Source: CAD feature listing. Evaluate the final solid. Frame: model axes, mm. A direction names the side the tool comes from. Round coordinates to 2 decimals unless told otherwise and drop trailing zeros. Loops run counter-clockwise (first coordinate to the right, second up) from the corner with the lowest first, then second, coordinate; pieces in that order, holes last. Notation, with made-up numbers: M 60.5,2.5 L 105.5,2.5 A25 cw 105.5,29.5 Z; hole C 79,24.25 d8. An arc over 180 degrees is marked long. One line per item, written item: value.
from build123d import *

# Parameters (mm, degrees)
SALIENTE_EXTRUIR1_DEPTH = 50.8
CROQUIS2_R              = 6.5
CORTAR_EXTRUIR1_DEPTH   = 10
CROQUIS3_R              = 6.5
CORTAR_EXTRUIR2_DEPTH   = 10


with BuildPart() as part:
    # Croquis1 → Saliente-Extruir1 (new body)
    with BuildSketch(Plane(origin=(0, 0, 0), x_dir=(0, 0, -1), z_dir=(1, 0, 0))):
        Polygon((-6.31, 95.93), (0, 95.93), (0, 0), (-902.2, 0), (-902.2, 6.31), (-6.31, 6.31), align=None)
    extrude(amount=SALIENTE_EXTRUIR1_DEPTH)

    # Croquis2 → Cortar-Extruir1 (cut)
    with BuildSketch(Plane(origin=(0, 0, 0), x_dir=(-1, 0, 0), z_dir=(0, -1, 0))):
        with Locations(Location((-25.4, -885.7, 0), (0, 0, 90))):
            Circle(CROQUIS2_R)
        with Locations(Location((-25.4, -854.7, 0), (0, 0, 90))):
            Circle(CROQUIS2_R)
    extrude(amount=-CORTAR_EXTRUIR1_DEPTH, mode=Mode.SUBTRACT)

    # Croquis3 → Cortar-Extruir2 (cut)
    with BuildSketch(Plane(origin=(0, 0, 0), x_dir=(-1, 0, 0), z_dir=(0, 0, -1))):
        with Locations(Location((-25.4, 70.53, 0), (0, 0, 90))):
            Circle(CROQUIS3_R)
    extrude(amount=-CORTAR_EXTRUIR2_DEPTH, mode=Mode.SUBTRACT)


solid = part.part
1. Section query B-B (y = 56). Return the cut outline in (x, z), and give its area (3 significant figures).
Report:
outline: M 0,0 L 50.8,0 L 50.8,6.31 L 0,6.31 Z
area: 321 mm2
2. Section query A-A (x = 11). Return the cut outline in (y, z).
Report:
outline: M 0,0 L 95.93,0 L 95.93,6.31 L 6.31,6.31 L 6.31,902.2 L 0,902.2 Z
3. Ray query, line 1 (Z direction, x = 25, y = 5); line 2 (Y direction, x = 25, z = 3); line 3 (X direction, y = 70, z = 1). Return the intervals inside material, ascending. Write a range as [from, to].
Report:
line 1: z = [0, 848.21], [861.19, 879.21], [892.19, 902.2]
line 2: y = [0, 64.04], [77.02, 95.93]
line 3: x = [0, 18.92], [31.88, 50.8]
4. Reachability of faces 1 (the face through (50.8, 6, 449)), 2 (the face through (25, 6.31, 461)) from +Z, -Z, +X, -X, +Y, -Y: full face, straight path, thin tool, end or side. Return the list, or none.
Report:
face 1: +Z, -Z, +X, +Y, -Y
face 2: +Z, +X, -X, +Y
5. Pin query (flat end, axial travel): pin 1 (5 mm diameter, centred on x = 41, z = 168.5, fed in from -Y). Return the tip coordinate at first contact, or that it passes through.
Report:
pin 1: stops at y = 0
